```python
from build123d import *

# Parameters (mm, degrees)
BOSS_EXTRUDE2_DEPTH     = 5
BOSS_EXTRUDE3_DEPTH     = 5
BOSS_EXTRUDE4_DEPTH     = 4.5
CHAMFER1_SIZE           = 3
BOSS_EXTRUDE5_DEPTH     = 11.5
BOSS_EXTRUDE6_DEPTH     = 11.5
FILLET2_R               = 1
SKETCH11_W              = 8
SKETCH11_H              = 24
CUT_EXTRUDE6_DEPTH      = 67.666204955
CUT_EXTRUDE7_START      = -1
CUT_EXTRUDE7_DEPTH      = 67.488020314
CUT_EXTRUDE8_DEPTH      = 8
FILLET3_R               = 1
CHAMFER9_SIZE           = 1
CUT_EXTRUDE9_DEPTH      = 67.666205085
CUT_EXTRUDE9_DEPTH_BACK = 67.666205085
SKETCH14_R              = 1.75
CHAMFER10_SIZE          = 2
CHAMFER8_SIZE           = 3
SKETCH16_W              = 5.209820602
SKETCH16_H              = 27.835500312
CUT_EXTRUDE10_DEPTH     = 67.666205085
CUT_EXTRUDE11_REACH     = 75.086
SKETCH17_R              = 2
CHAMFER12_SIZE          = 0.5
CHAMFER12_SIZE2         = 0.866025404


with BuildPart() as part:
    # Sketch1 → Boss-Extrude2 (new body)
    with BuildSketch(Plane(origin=(0, 0, 0), x_dir=(1, 0, 0), z_dir=(0, 1, 0))):
        Polygon((-32.851435656, 19.25), (14.148564344, 19.25), (14.148564344, 15), (-1.351435656, 15), (-1.351435656, -15), (14.148564344, -15), (14.148564344, -19.25), (-32.851435656, -19.25), (-32.851435656, -35), (22.148564344, -35), (22.148564344, 35), (-32.851435656, 35), align=None)
    extrude(amount=BOSS_EXTRUDE2_DEPTH)

    # Sketch5 → Boss-Extrude3 (add)
    with BuildSketch(Plane(origin=(0, 5, 0), x_dir=(1, 0, 0), z_dir=(0, 1, 0))):
        Polygon((-32.851435656, 35), (22.148564344, 35), (22.148564344, -35), (-32.851435656, -35), (-32.851435656, -23.5), (14.148564344, -23.5), (14.148564344, -15), (-1.351435656, -15), (-1.351435656, 15), (14.148564344, 15), (14.148564344, 23.5), (-32.851435656, 23.5), align=None)
    extrude(amount=BOSS_EXTRUDE3_DEPTH)

    # Sketch6 → Boss-Extrude4 (add)
    with BuildSketch(Plane(origin=(0, 10, 0), x_dir=(1, 0, 0), z_dir=(0, 1, 0))):
        with BuildLine():
            Line((22.148564344, 35), (-46.851435656, 35))
            Line((-46.851435656, 35), (-46.851435656, 20))
            Line((-46.851435656, 20), (-54.851435656, 16))
            add(Edge.make_bspline(
                [(-54.851435656, -16), (-56.851435656, 0), (-54.851435656, 16)],
                knots=[0, 0, 0, 1, 1, 1], degree=2))
            Line((-54.851435656, -16), (-46.851435656, -20))
            Line((-46.851435656, -20), (-46.851435656, -35))
            Line((-46.851435656, -35), (22.148564344, -35))
            Line((22.148564344, -35), (22.148564344, -23))
            Line((22.148564344, -23), (22.148564344, 23))
            Line((22.148564344, 23), (22.148564344, 35))
        make_face()
    extrude(amount=BOSS_EXTRUDE4_DEPTH)

    # Chamfer1
    chamfer1_edges = [part.edges().sort_by_distance(p)[0] for p in [
        (-46.851435656, 10, -27.5),
        (-46.851435656, 10, 27.5),
    ]]
    chamfer(chamfer1_edges, length=CHAMFER1_SIZE)

    # Sketch7 → Boss-Extrude5 (add)
    with BuildSketch(Plane.XY.offset(35)):
        Polygon((-33.851435656, 0), (-43.851435656, 10), (-32.851435656, 10), (-32.851435656, 0), align=None)
    extrude(amount=-BOSS_EXTRUDE5_DEPTH)

    # Sketch8 → Boss-Extrude6 (add)
    with BuildSketch(Plane(origin=(0, 0, -35), x_dir=(-1, 0, 0), z_dir=(0, 0, -1))):
        Polygon((43.851435656, 10), (33.851435656, 0), (32.851435656, 0), (32.851435656, 10), align=None)
    extrude(amount=-BOSS_EXTRUDE6_DEPTH)

    # Fillet2
    fillet2_edges = [part.edges().sort_by_distance(p)[0] for p in [
        (-5.851435656, 0, -35),
        (22.148564344, 0, 0),
        (-5.851435656, 0, 35),
        (-9.351435656, 0, 19.25),
        (-1.351435656, 0, 0),
        (-9.351435656, 0, -19.25),
        (22.148564344, 7.25, -35),
        (22.148564344, 7.25, 35),
        (-1.351435656, 5, 15),
        (-1.351435656, 5, -15),
        (-9.351435656, 5, 19.25),
        (-9.351435656, 5, -19.25),
    ]]
    fillet(fillet2_edges, radius=FILLET2_R)

    # Sketch11 → Cut-Extrude6 (cut, through all)
    with BuildSketch(Plane.XZ.offset(-10)):
        with Locations((-47.851435656, 0)):
            Rectangle(SKETCH11_W, SKETCH11_H)
    extrude(amount=-CUT_EXTRUDE6_DEPTH, mode=Mode.SUBTRACT)

    # Sketch12 → Cut-Extrude7 (cut, through all)
    with BuildSketch(Plane.XZ.offset(CUT_EXTRUDE7_START)):
        Polygon((8.648564344, 13.5), (20.148564344, 13.5), (20.148564344, -13.5), (8.648564344, -13.5), (8.648564344, -7), (8.648564344, 7), align=None)
    extrude(amount=-CUT_EXTRUDE7_DEPTH, mode=Mode.SUBTRACT)

    # Sketch13 → Cut-Extrude8 (cut)
    with BuildSketch(Plane.ZY.offset(1.351435656)):
        with BuildLine():
            Line((11.4, 2.171572875), (11.4, 2.25))
            Line((11.4, 2.25), (12.6, 2.25))
            Line((12.6, 2.25), (12.6, 8.75))
            Line((12.6, 8.75), (11.4, 8.75))
            Line((11.4, 8.75), (11.4, 7.5))
            Line((11.4, 7.5), (10.9, 7.5))
            ThreePointArc((10.9, 7.5), (9.052240935, 6.265366865), (9.485786438, 4.085786438))
            Line((9.485786438, 4.085786438), (11.4, 2.171572875))
        make_face()
        with BuildLine():
            Line((-12.6, 8.75), (-11.4, 8.75))
            Line((-11.4, 8.75), (-11.4, 7.5))
            Line((-11.4, 7.5), (-10.9, 7.5))
            ThreePointArc((-10.9, 7.5), (-9.052240935, 6.265366865), (-9.485786438, 4.085786438))
            Line((-9.485786438, 4.085786438), (-11.4, 2.171572875))
            Line((-11.4, 2.171572875), (-11.4, 2.25))
            Line((-11.4, 2.25), (-12.6, 2.25))
            Line((-12.6, 2.25), (-12.6, 8.75))
        make_face()
    extrude(amount=-CUT_EXTRUDE8_DEPTH, mode=Mode.SUBTRACT)

    # Fillet3
    fillet3_edges = [part.edges().sort_by_distance(p)[0] for p in [
        (-49.351435656, 10, -18.75),
        (-55.851435656, 10, 0),
        (-49.351435656, 10, 18.75),
    ]]
    fillet(fillet3_edges, radius=FILLET3_R)

    # Chamfer9
    chamfer9_edges = [part.edges().sort_by_distance(p)[0] for p in [
        (-51.851435656, 10, 0),
        (-47.851435656, 10, -12),
        (-43.851435656, 10, 0),
        (-47.851435656, 10, 12),
    ]]
    chamfer(chamfer9_edges, length=CHAMFER9_SIZE)

    # Sketch14 → Cut-Extrude9 (cut, two sides: drawn at the far end of the back side and taken through both)
    with BuildSketch(Plane.XZ.offset(-10).offset(-CUT_EXTRUDE9_DEPTH_BACK)):
        with Locations(Location((-32.851435656, 15, 0), (0, 0, 270))):
            Circle(SKETCH14_R)
        with Locations(Location((-32.851435656, -15, 0), (0, 0, 270))):
            Circle(SKETCH14_R)
        with Locations((27.148564344, -15)):
            Circle(SKETCH14_R)
        with Locations((27.148564344, 15)):
            Circle(SKETCH14_R)
        with Locations(Location((7.148564344, 28, 0), (0, 0, 270))):
            Circle(SKETCH14_R)
        with Locations(Location((7.148564344, -28, 0), (0, 0, 270))):
            Circle(SKETCH14_R)
    extrude(amount=CUT_EXTRUDE9_DEPTH + CUT_EXTRUDE9_DEPTH_BACK, mode=Mode.SUBTRACT)

    # Chamfer10
    chamfer10_edges = [part.edges().sort_by_distance(p)[0] for p in [
        (7.148564344, 0, -26.25),
        (-32.851435656, 10, -13.25),
        (7.148564344, 0, 29.75),
        (-32.851435656, 10, 16.75),
    ]]
    chamfer(chamfer10_edges, length=CHAMFER10_SIZE)

    # Chamfer8
    # the kernel refuses this chamfer: 3 mm, written as the material it takes off along each edge
    with BuildSketch(Plane(origin=(-32.851435656, -6.715048964, -19.25), x_dir=(0.9996219169112965, 0, 0.02749587661058676), z_dir=(0, 1, 0))) as chamfer8_piece_1_section:
        Polygon((CHAMFER8_SIZE * 0.999621916911, CHAMFER8_SIZE * 0.0274958766106), (-CHAMFER8_SIZE * 0.0274958766106, CHAMFER8_SIZE * 0.999621916911), (0, 0), align=None)
    chamfer8_piece_1 = extrude(amount=18.430097928, mode=Mode.PRIVATE)
    chamfer8_piece_1 = split(chamfer8_piece_1, bisect_by=Plane(origin=(-31.873507714, 5, -20.294144115), z_dir=(0, -1, 0)), keep=Keep.TOP, mode=Mode.PRIVATE)
    add(chamfer8_piece_1, mode=Mode.SUBTRACT)
    with BuildSketch(Plane(origin=(-32.851435656, -6.715048964, 19.25), x_dir=(0.9996219169112968, 0, -0.027495876610586733), z_dir=(0, 1, 0))) as chamfer8_piece_2_section:
        Polygon((CHAMFER8_SIZE * 0.999621916911, -CHAMFER8_SIZE * 0.0274958766106), (-CHAMFER8_SIZE * 0.0274958766106, -CHAMFER8_SIZE * 0.999621916911), (0, 0), align=None)
    chamfer8_piece_2 = extrude(amount=18.430097928, mode=Mode.PRIVATE)
    chamfer8_piece_2 = split(chamfer8_piece_2, bisect_by=Plane(origin=(-31.873507712, 5, 20.294144115), z_dir=(0, -1, 0)), keep=Keep.TOP, mode=Mode.PRIVATE)
    add(chamfer8_piece_2, mode=Mode.SUBTRACT)

    # Sketch16 → Cut-Extrude10 (cut, through all)
    with BuildSketch(Plane.XZ.offset(-10)):
        with Locations((-3.956345957, 0.082249844)):
            Rectangle(SKETCH16_W, SKETCH16_H)
    extrude(amount=-CUT_EXTRUDE10_DEPTH, mode=Mode.SUBTRACT)

    # Sketch17 → Cut-Extrude11 (cut, up to next)
    with BuildSketch(Plane.ZY.offset(-6.648564344), mode=Mode.PRIVATE) as cut_extrude11_sk1:
        with Locations((-10.9, 5.5)):
            Circle(SKETCH17_R)
    cut_extrude11_tool1 = extrude(cut_extrude11_sk1.sketch, amount=-CUT_EXTRUDE11_REACH, mode=Mode.PRIVATE) & part.part
    # Sketch17 → Cut-Extrude11 (cut, up to next)
    with BuildSketch(Plane.ZY.offset(-6.648564344), mode=Mode.PRIVATE) as cut_extrude11_sk2:
        with Locations((10.9, 5.5)):
            Circle(SKETCH17_R)
    cut_extrude11_tool2 = extrude(cut_extrude11_sk2.sketch, amount=-CUT_EXTRUDE11_REACH, mode=Mode.PRIVATE) & part.part
    add(cut_extrude11_tool1.solids().sort_by_distance((6.648564, 5.5, -10.9))[0], mode=Mode.SUBTRACT)
    add(cut_extrude11_tool2.solids().sort_by_distance((6.648564, 5.5, 10.9))[0], mode=Mode.SUBTRACT)

    # Chamfer12
    chamfer12_edges = [part.edges().sort_by_distance(p)[0] for p in [
        (8.648564344, 5.5, -12.9),
        (8.648564344, 5.5, 8.9),
    ]]
    chamfer12_side = [part.faces().sort_by_distance(p)[0] for p in [
        (8.648564344, 7.91662971, 0),
    ]]
    chamfer(chamfer12_edges, length=CHAMFER12_SIZE, length2=CHAMFER12_SIZE2, reference=chamfer12_side[0])


solid = part.part
```
Design review of the part built by this model. Coordinates are the model's own, in mm. A direction names the side the tool comes from. Coordinates: 2 decimals unless noted, no trailing zeros. Loops run counter-clockwise (first coordinate to the right, second up) from the corner with the lowest first, then second, coordinate; pieces in that order, holes last. Notation, with made-up numbers: M -22.5,36 L -7.5,36 A17 cw -7.5,63 Z; hole C -36,73.5 d6. An arc over 180 degrees is marked long. One line per question, with ' | ' between items.
(1) Machinability: for faces 1 (the face through (-43.851, 13, 0)), 2 (the face through (-8, 2, 19.25)), 3 (the face through (20.149, 8, 0)), 4 (the face through (3, 5, -12.6)), which of the approach directions +Z, -Z, +X, -X, +Y, -Y give a long, thin tool a straight path to every point of the face, cutting with its end or side? Answer none if there is none.
Filled in:
face 1: +Y, -Y | face 2: -X, -Y | face 3: +Y | face 4: -X
(2) We need section B-B (x = 16). Give the boundary of the cut face in (y, z), and give its area (3 significant figures).
Filled in:
outline: M 0,-34 A1 ccw 1,-35 L 14.5,-35 L 14.5,-13.5 L 1,-13.5 L 1,13.5 L 14.5,13.5 L 14.5,35 L 1,35 A1 ccw 0,34 Z | area: 650 mm^2
(3) We need section A-A (z = -28). Give the boundary of the cut face in (x, y).
Filled in:
outline: M -46.85,13 L -33.85,0 L 3.4,0 L 5.4,2 L 5.4,14.5 L -46.85,14.5 Z; M 8.9,2 L 10.9,0 L 21.15,0 A1 ccw 22.15,1 L 22.15,14.5 L 8.9,14.5 Z
(4) Draft analysis for pull direction X (two halves, no side actions). For faces 5 (the face through (14, 8, 13.5)), 6 (the face through (22.149, 8, 0)), 7 (the face through (-13, 8, -35)), 8 (the face through (-40.44, 6.59, -29.27)), state which applies: released by +X, released by -X, zero draft, split by the parting line, or undercut.
Filled in:
face 5: undercut | face 6: released by +X | face 7: zero draft | face 8: released by -X
(5) Wall thickness on probe 1 along Z at (x, y) = (-8, 9); probe 2 along X at (y, z) = (1.75, -11.5); probe 3 along Y at (x, z) = (-14, 22): over which ranges is each line inside the solid? List them lowest first.
Filled in:
probe 1: z = -35 to -23.5, 23.5 to 35 | probe 2: x = -1.35 to 8.65, 20.15 to 22.15 | probe 3: y = 0 to 5, 10 to 14.5
(6) For pin 1 Ø5 at (x, z) = (-36.5, 17.5) entering from -Y; pin 2 Ø8 at (y, z) = (7, 14) entering from -X; pin 3 Ø5.5 at (x, z) = (7.15, -28) entering from +Y; pin 4 Ø1 at (x, y) = (-48, 13) entering from +Z, all flat-tipped, find the tip position at first contact; note any pin that passes through.
Filled in:
pin 1: stops at y = 10 | pin 2: stops at x = -55.2 | pin 3: stops at y = 14.5 | pin 4: stops at z = 19.68
(7) We need section C-C (x = -14). Give the boundary of the cut face in (y, z), and give its area (3 significant figures).
Filled in:
outline: M 0,-34 A1 ccw 1,-35 L 14.5,-35 L 14.5,35 L 1,35 A1 ccw 0,34 L 0,20.25 A1 ccw 1,19.25 L 4,19.25 A1 ccw 5,20.25 L 5,23.5 L 10,23.5 L 10,-23.5 L 5,-23.5 L 5,-20.25 A1 ccw 4,-19.25 L 1,-19.25 A1 ccw 0,-20.25 Z | area: 586 mm^2
